Read the model definition and answer for the solid it produces. Units are mm, in the model's axes. Face numbers are marked on the shaded views. A direction names the side the tool comes from. Give positions to 0.01 mm unless a question says otherwise; leave off trailing zeros. Order: outer loops, then holes, each group sorted by start corner. A loop starts at its lowest first (then second) coordinate and runs counter-clockwise, first axis right, second up. Notation, with made-up numbers: (35, -10) -> (55, -10) arc R26 ccw to (55, 20) -> close; hole circle Ø6 at (-3.5, 55.5). An arc over 180 degrees is marked (long way). Use one line per item in the form item = value.
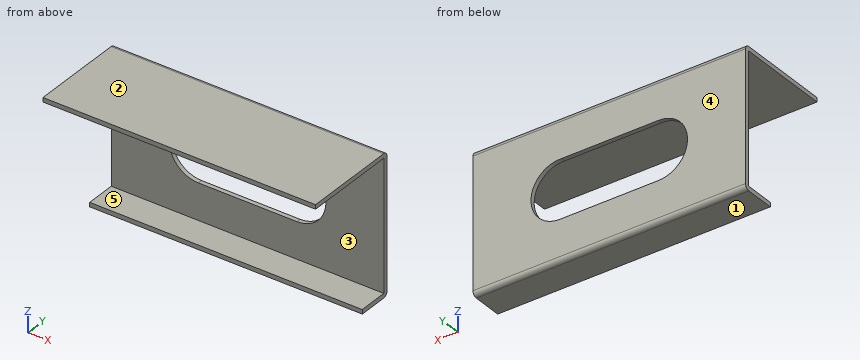
```python
from build123d import *

# Parameters (mm, degrees)
F1_DEPTH = 298.45
F2_R     = 5.08
F4_D     = 63.5
F6_DEPTH = 25.4


with BuildPart() as f1:
    # F0 (on Right) → F1 (new body)
    with BuildSketch(Plane.YZ):
        Polygon((0, -85.7519404639), (0, 66.6480595361), (-107.95, 66.6480595361), (-107.95, 61.8728595361), (-4.7752, 61.8728595361), (-4.7752, -80.9767404639), (-37.338, -80.9767404639), (-37.338, -85.7519404639), align=None)
    extrude(amount=F1_DEPTH)

    # F2
    f2_edges = [f1.edges().sort_by_distance(p)[0] for p in [
        (149.225, 0, 66.64806),
        (149.225, 0, -85.75194),
    ]]
    fillet(f2_edges, radius=F2_R)

    # F4 (through all)
    with Locations(Plane(origin=(0, 0, 0), x_dir=(-1, 0, 0), z_dir=(0, 1, 0))):
        with Locations((-203.2, -9.5519404639), (-95.25, -9.5519404639)):
            Hole(F4_D / 2)

    # F5 (on face) → F6 (cut)
    with BuildSketch(Plane(origin=(0, 0, 0), x_dir=(-1, 0, 0), z_dir=(0, 1, 0))):
        with BuildLine():
            Line((-95.2632086497, 22.1980567886), (-201.5250755989, 22.1538496737))
            ThreePointArc((-201.5250755989, 22.1538496737), (-180.1647948812, 12.2985017543), (-171.45, -9.5519404639))
            ThreePointArc((-171.45, -9.5519404639), (-180.7493594116, -32.0025804808), (-203.1999991918, -41.3019404639))
            Line((-203.1999991918, -41.3019404639), (-95.2632086497, -41.3019377164))
            ThreePointArc((-95.2632086497, -41.3019377164), (-127, -9.5519404639), (-95.2632086497, 22.1980567886))
        make_face()
    extrude(amount=-F6_DEPTH, mode=Mode.SUBTRACT)


solid = f1.part
```
Item 1: The part is cut by section A-A on y = -19. Give the vertices of the cut face in (x, z), and give its area (3 significant figures).
Checks:
outline = (0, -85.75) -> (298.45, -85.75) -> (298.45, -80.98) -> (0, -80.98) -> close; (0, 61.87) -> (298.45, 61.87) -> (298.45, 66.65) -> (0, 66.65) -> close
area = 2,850 mm²
Item 2: Given pin 1 Ø4 at (x, z) = (209.5, -82.5) entering from -Y; pin 2 Ø12 at (x, z) = (53.5, -22) entering from -Y; pin 3 Ø1.4 at (x, y) = (126.5, -3) entering from +Z, each flat-ended and moving along its own axis, determine where each tip first touches the part or whether it passes through.
Checks:
pin_1 = -37.34
pin_2 = -4.78
pin_3 = 66.46
Item 3: The part is cut by section C-C on x = 138.5. Give the vertices of the cut face in (y, z), and give its area (3 significant figures).
Checks:
outline = (-107.95, 61.87) -> (-4.78, 61.87) -> (-4.78, 22.18) -> (0, 22.18) -> (0, 61.57) arc R5.08 ccw to (-5.08, 66.65) -> (-107.95, 66.65) -> close; (-37.34, -85.75) -> (-5.08, -85.75) arc R5.08 ccw to (0, -80.67) -> (0, -41.3) -> (-4.78, -41.3) -> (-4.78, -80.98) -> (-37.34, -80.98) -> close
area = 1,060 mm²
Item 4: Straight lines are drawn through the part: L1, parallel to Z at x = 52.5, y = -18; L2, parallel to Y at x = 88, z = -45; L3, parallel to Z at x = 151, y = -70.5. For each, find the intervals that lie inside material, in ascending order. Write a range as from..to.
Checks:
L1 = -85.75..-80.98, 61.87..66.65
L2 = -4.78..0
L3 = 61.87..66.65
Item 5: The part is cut by section D-D on z = -67.5. Give the vertices of the cut face in (x, y), and give its area (3 significant figures).
Checks:
outline = (0, -4.78) -> (298.45, -4.78) -> (298.45, 0) -> (0, 0) -> close
area = 1,430 mm²
Item 6: Which of the six approach directions +Z, -Z, +X, -X, +Y, -Y give full straight-line access (tool end or side, diameter ignored) to the marked faces 4 and 5?
Checks:
face_4 = +Z, -Z, +X, -X, +Y
face_5 = +X, -X, -Y
Item 7: Determine the mould class of the marked faces 1, 2 and 3 for opening direction Z: +Z half, -Z half, draft (parallel to the pull), parting line (faces both ways), or undercut.
Checks:
face_1 = -Z half
face_2 = +Z half
face_3 = undercut
Item 8: The part is cut by section B-B on x = 266.5. Give the vertices of the cut face in (y, z), and give its area (3 significant figures).
Checks:
outline = (-107.95, 61.87) -> (-4.78, 61.87) -> (-4.78, -80.98) -> (-37.34, -80.98) -> (-37.34, -85.75) -> (-5.08, -85.75) arc R5.08 ccw to (0, -80.67) -> (0, 61.57) arc R5.08 ccw to (-5.08, 66.65) -> (-107.95, 66.65) -> close
area = 1,360 mm²
